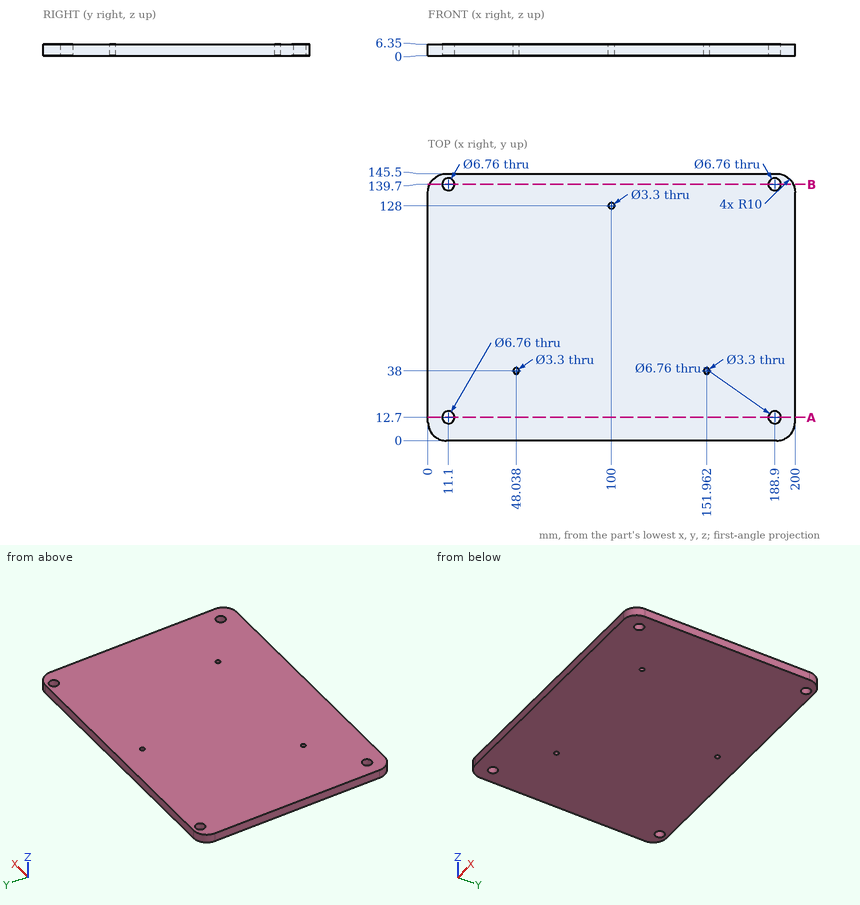
Here's the drawing with two shaded views (mm, measured from the low corner). I have some questions. Coordinates: 2 decimals unless noted, no trailing zeros. Order: outer loops, then holes, each group sorted by start corner. A loop starts at its lowest first (then second) coordinate and runs counter-clockwise, first axis right, second up.
Q1. Please list where these lines run through material, in increasing order: L1, parallel to Y at x = 11.1, z = 3; L2, parallel to Y at x = 100, z = 3.25; L3, parallel to X at y = 138, z = 2.25.
Q2. Suppose I cut it at A-A on y = 12.7. Please give me the cut outline in (x, z), and give its area (3 significant figures).
Q3. Suppose I cut it at B-B on y = 139.7. Give the number of separate pieces and of enclosed holes in the cut face, and give its area (3 significant figures).
Answer:
1. L1: y = 0 to 9.32, 16.08 to 136.32, 143.08 to 145.5
1. L2: y = 0 to 126.35, 129.65 to 145.5
1. L3: x = 0.32 to 8.18, 14.02 to 185.98, 191.82 to 199.68
2. outline: (0, 0) - (7.72, 0) - (7.72, 6.35) - (0, 6.35) - close; (14.48, 0) - (185.52, 0) - (185.52, 6.35) - (14.48, 6.35) - close; (192.28, 0) - (200, 0) - (200, 6.35) - (192.28, 6.35) - close
2. area: 1,180 mm2
3. separate pieces: 3
3. enclosed holes: 0
3. area: 1,170 mm2
